```python
from build123d import *

# Parameters (mm, degrees)
SKETCH1_W             = 70
SKETCH1_H             = 30
SKETCH1_R             = 7
SKETCH1_R_2           = 1.495
SKETCH1_R_3           = 0.995
SKETCH1_R_4           = 2
BOSS_EXTRUDE1_DEPTH   = 6.35
F_2_CLEARANCE_HOLE1_D = 2.2606


with BuildPart() as part:
    # Sketch1 → Boss-Extrude1 (new body)
    with BuildSketch(Plane.XY):
        with Locations((20, 0)):
            Rectangle(SKETCH1_W, SKETCH1_H)
        Circle(SKETCH1_R, mode=Mode.SUBTRACT)
        with Locations((18.05, 0)):
            Circle(SKETCH1_R_2, mode=Mode.SUBTRACT)
        with Locations((32.6, 0)):
            Circle(SKETCH1_R_3, mode=Mode.SUBTRACT)
        with Locations((42.449999958, 0)):
            Circle(SKETCH1_R_4, mode=Mode.SUBTRACT)
    extrude(amount=BOSS_EXTRUDE1_DEPTH)

    # #2 Clearance Hole1 (through all)
    with Locations(Plane.XY.offset(6.35)):
        with Locations((-12.5, 12.5), (-12.5, -12.5), (27.5, 12.5), (27.5, -12.5), (52.5, 12.5), (52.5, -12.5)):
            Hole(F_2_CLEARANCE_HOLE1_D / 2)


solid = part.part
```
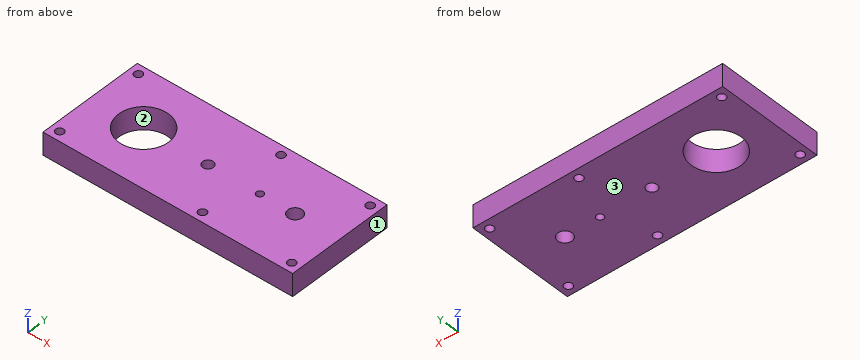
Part model, mm, in its own coordinate system. Face numbers are marked on the shaded views. Coordinates: 2 decimals unless noted, no trailing zeros. Loops run counter-clockwise (first coordinate to the right, second up) from the corner with the lowest first, then second, coordinate; pieces in that order, holes last. Notation, with made-up numbers: (22.25, 84) - (72.25, 84) arc R26 ccw to (72.25, 114) - close; hole circle Ø1 at (34, 67). An arc over 180 degrees is marked (long way). Write item = value, one per line. Start each with the question number.
Item 1: Wall check: L1, parallel to Y at x = 52.5, z = 4; L2, parallel to Y at x = 32.6, z = 1.75 (3 decimals); L3, parallel to X at y = 12, z = 0.5. Give the ranges that are in metal, low to high. Write a range as from..to.
Item 2: Mould opens along X. For the marked faces 1, 2 and 3 say: released by +X, released by -X, zero draft, split by the parting line, or undercut.
Item 3: Cut at B-B, the plane y = 0. Give the cut face in (x, z) (3 decimals), and give its area (3 significant figures).
Item 4: Cut at A-A, the plane x = 18.05. Give the cut face in (y, z) (3 decimals).
Item 5: Cut at C-C, the plane x = 27.5. Give the cut face in (y, z).
Item 6: Cut at D-D, the plane z = 1.75. State how many separate pieces and enclosed holes the cut face has, and give its area (3 significant figures).
The answers:
q1.L1 = -15..-13.63, -11.37..11.37, 13.63..15
q1.L2 = -15..-0.995, 0.995..15
q1.L3 = -15..-13.51, -11.49..26.49, 28.51..51.49, 53.51..55
q2.face_1 = released by +X
q2.face_2 = undercut
q2.face_3 = zero draft
q3.outline = (-15, 0) - (-7, 0) - (-7, 6.35) - (-15, 6.35) - close; (7, 0) - (16.555, 0) - (16.555, 6.35) - (7, 6.35) - close; (19.545, 0) - (31.605, 0) - (31.605, 6.35) - (19.545, 6.35) - close; (33.595, 0) - (40.45, 0) - (40.45, 6.35) - (33.595, 6.35) - close; (44.45, 0) - (55, 0) - (55, 6.35) - (44.45, 6.35) - close
q3.area = 299 mm2
q4.outline = (-15, 0) - (-1.495, 0) - (-1.495, 6.35) - (-15, 6.35) - close; (1.495, 0) - (15, 0) - (15, 6.35) - (1.495, 6.35) - close
q5.outline = (-15, 0) - (-13.63, 0) - (-13.63, 6.35) - (-15, 6.35) - close; (-11.37, 0) - (11.37, 0) - (11.37, 6.35) - (-11.37, 6.35) - close; (13.63, 0) - (15, 0) - (15, 6.35) - (13.63, 6.35) - close
q6.separate_pieces = 1
q6.enclosed_holes = 10
q6.area = 1,900 mm2
